Design review of the part built by this model. Coordinates are the model's own, in mm. Face numbers are marked on the shaded views. A direction names the side the tool comes from. Coordinates: 2 decimals unless noted, no trailing zeros. Order: outer loops, then holes, each group sorted by start corner. A loop starts at its lowest first (then second) coordinate and runs counter-clockwise, first axis right, second up. Notation, with made-up numbers: M 28.25,-24.75 L 70.25,-24.75 A16 cw 70.25,-20.75 Z; hole C -4.5,6 d1. An arc over 180 degrees is marked long. Use CSV: the item, a comma, the result in double quotes.
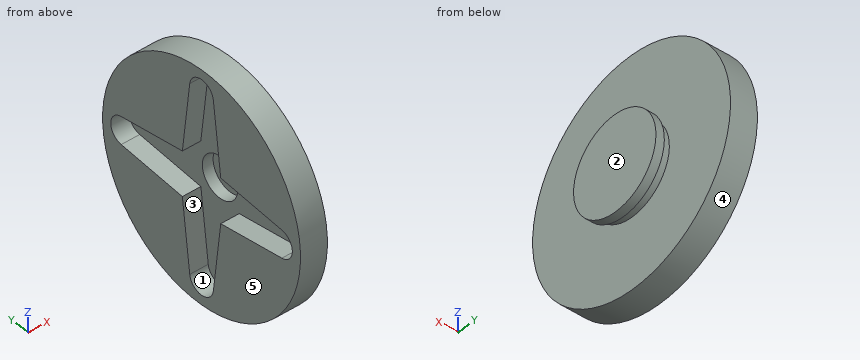
```python
from build123d import *

# Parameters (mm, degrees)
SKETCH2_R           = 33.5
BOSS_EXTRUDE1_DEPTH = 8
SKETCH7_R           = 12.8
BOSS_EXTRUDE2_DEPTH = 2.5
SKETCH8_R           = 13.95
BOSS_EXTRUDE3_DEPTH = 2.5
CUT_EXTRUDE1_DEPTH  = 5.5
SKETCH11_R          = 6
CUT_EXTRUDE2_DEPTH  = 3.2


with BuildPart() as part:
    # Sketch2 → Boss-Extrude1 (new body)
    with BuildSketch(Plane(origin=(0, 0, 0), x_dir=(0, 0, -1), z_dir=(1, 0, 0))):
        Circle(SKETCH2_R)
    extrude(amount=BOSS_EXTRUDE1_DEPTH)

    # Sketch7 → Boss-Extrude2 (add)
    with BuildSketch(Plane(origin=(8, 0, 0), x_dir=(0, 0, -1), z_dir=(1, 0, 0))):
        Circle(SKETCH7_R)
    extrude(amount=BOSS_EXTRUDE2_DEPTH)

    # Sketch8 → Boss-Extrude3 (add)
    with BuildSketch(Plane(origin=(10.5, 0, 0), x_dir=(0, 0, -1), z_dir=(1, 0, 0))):
        Circle(SKETCH8_R)
    extrude(amount=BOSS_EXTRUDE3_DEPTH)

    # Sketch10 → Cut-Extrude1 (cut)
    with BuildSketch(Plane.ZY):
        with BuildLine():
            Line((-4, -27.203944189), (-6.5, -6.5))
            Line((-6.5, -6.5), (-27.203944189, -4))
            ThreePointArc((-27.203944189, -4), (-30.75, 0), (-27.203944189, 4))
            Line((-27.203944189, 4), (-6.5, 6.5))
            Line((-6.5, 6.5), (-4, 27.203944189))
            ThreePointArc((-4, 27.203944189), (0, 30.75), (4, 27.203944189))
            Line((4, 27.203944189), (6.5, 6.5))
            Line((6.5, 6.5), (27.203944189, 4))
            ThreePointArc((27.203944189, 4), (30.75, 0), (27.203944189, -4))
            Line((27.203944189, -4), (6.5, -6.5))
            Line((6.5, -6.5), (4, -27.203944189))
            ThreePointArc((4, -27.203944189), (0, -30.75), (-4, -27.203944189))
        make_face()
    extrude(amount=-CUT_EXTRUDE1_DEPTH, mode=Mode.SUBTRACT)

    # Sketch11 → Cut-Extrude2 (cut)
    with BuildSketch(Plane.ZY.offset(-5.5)):
        Circle(SKETCH11_R)
    extrude(amount=-CUT_EXTRUDE2_DEPTH, mode=Mode.SUBTRACT)


solid = part.part
```
(1) Add section D-D on z = 10. State the section outline as (x, y) points, and give its area (3 significant figures).
The answers:
outline,"M 0,-31.97 L 8,-31.97 L 8,-7.99 L 10.5,-7.99 L 10.5,-9.73 L 13,-9.73 L 13,9.73 L 10.5,9.73 L 10.5,7.99 L 8,7.99 L 8,31.97 L 0,31.97 L 0,6.08 L 5.5,6.08 L 5.5,-6.08 L 0,-6.08 Z"
area,"533 mm2"
(2) Add section B-B on z = 0. State the section outline as (x, y) points.
The answers:
outline,"M 0,-33.5 L 8,-33.5 L 8,-12.8 L 10.5,-12.8 L 10.5,-13.95 L 13,-13.95 L 13,13.95 L 10.5,13.95 L 10.5,12.8 L 8,12.8 L 8,33.5 L 0,33.5 L 0,30.75 L 5.5,30.75 L 5.5,6 L 8.7,6 L 8.7,-6 L 5.5,-6 L 5.5,-30.75 L 0,-30.75 Z"
(3) Wall thickness on probe 1 along Y at (x, z) = (6.6, 0); probe 2 along X at (y, z) = (24, 16); probe 3 along Y at (x, z) = (1.5, 10): over which ranges is each line inside the solid? List them lowest first.
The answers:
probe 1,"y = -33.5 to -6, 6 to 33.5"
probe 2,"x = 0 to 8"
probe 3,"y = -31.97 to -6.08, 6.08 to 31.97"
(4) For the marked faces 1 and 2, list the 3-axis set-ups (+Z, -Z, +X, -X, +Y, -Y) from which the entire face can be reached by the end or side of a thin tool; tool diameter is ignored.
The answers:
face 1,"-X"
face 2,"+Z, -Z, +X, +Y, -Y"
(5) Add section A-A on x = 4. State the section outline as (y, z) points.
The answers:
outline,"C 0,0 d67; hole M -27.2,-4 L -6.5,-6.5 L -4,-27.2 A4.03 ccw 4,-27.2 L 6.5,-6.5 L 27.2,-4 A4.03 ccw 27.2,4 L 6.5,6.5 L 4,27.2 A4.03 ccw -4,27.2 L -6.5,6.5 L -27.2,4 A4.03 ccw Z"
(6) The part is to be moulded in two halves that separate along Y. For the marked faces 3, 4 and 5, say which applies: pulls with the +Y half, pulls with the -Y half, needs draft (parallel to the pull), parting line crosses it, or undercut.
The answers:
face 3,"undercut"
face 4,"parting line crosses it"
face 5,"needs draft"
(7) Clearance check with flat-ended pins moving along their axes: P1, Ø9.5, axis at y = 0, z = 0, coming from the -X side; P2, Ø2, axis at x = 5, y = -9, coming from the +Z side; P3, Ø18.5, axis at y = 2, z = 8, coming from the -X side; P4, Ø2, axis at x = 8, y = 24.5, coming from the +Z side. State where each tip first meets the part, or that it passes through.
The answers:
P1,"stops at x = 8.7"
P2,"stops at z = 32.53"
P3,"stops at x = 0"
P4,"stops at z = 23.87"
